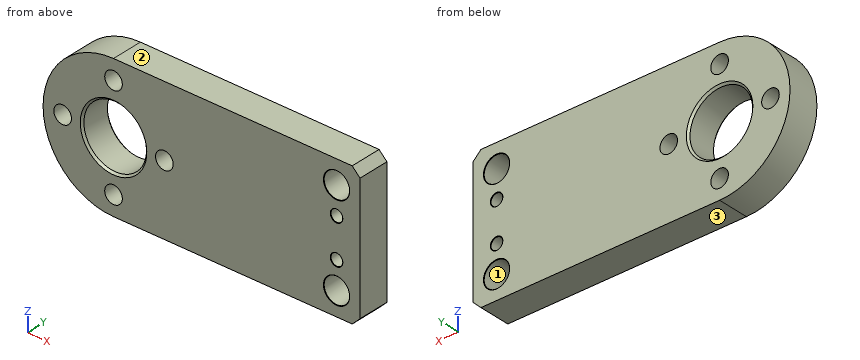
```python
from build123d import *

# Parameters (mm, degrees)
SKETCH1_R           = 8
SKETCH1_R_2         = 2.25
BOSS_EXTRUDE1_DEPTH = 8
SKETCH2_R           = 3.25
SKETCH2_R_2         = 1.5
CUT_EXTRUDE1_DEPTH  = 67.007575323
CHAMFER1_SIZE       = 0.5
CHAMFER2_SIZE       = 0.1


with BuildPart() as part:
    # Sketch1 → Boss-Extrude1 (new body)
    with BuildSketch(Plane(origin=(0, 0, 0), x_dir=(1, 0, 0), z_dir=(0, 1, 0))):
        with BuildLine():
            Line((0, 18), (61, 18))
            Line((61, 18), (63, 16))
            Line((63, 16), (63, -16))
            Line((63, -16), (61, -18))
            Line((61, -18), (0, -18))
            ThreePointArc((0, -18), (-18, 0), (0, 18))
        make_face()
        with Locations(Location((0, 0, 0), (0, 0, 270))):
            Circle(SKETCH1_R, mode=Mode.SUBTRACT)
        with Locations(Location((0, 13, 0), (0, 0, 270))):
            Circle(SKETCH1_R_2, mode=Mode.SUBTRACT)
        with Locations(Location((13, 0, 0), (0, 0, 270))):
            Circle(SKETCH1_R_2, mode=Mode.SUBTRACT)
        with Locations(Location((0, -13, 0), (0, 0, 270))):
            Circle(SKETCH1_R_2, mode=Mode.SUBTRACT)
        with Locations(Location((-13, 0, 0), (0, 0, 270))):
            Circle(SKETCH1_R_2, mode=Mode.SUBTRACT)
    extrude(amount=BOSS_EXTRUDE1_DEPTH)

    # Sketch2 → Cut-Extrude1 (cut, through all)
    with BuildSketch(Plane(origin=(0, 8, 0), x_dir=(1, 0, 0), z_dir=(0, 1, 0))):
        with Locations(Location((57, 12, 0), (0, 0, 270))):
            Circle(SKETCH2_R)
        with Locations(Location((57, 5, 0), (0, 0, 270))):
            Circle(SKETCH2_R_2)
        with Locations(Location((57, -5, 0), (0, 0, 90))):
            Circle(SKETCH2_R_2)
        with Locations(Location((57, -12, 0), (0, 0, 90))):
            Circle(SKETCH2_R)
    extrude(amount=-CUT_EXTRUDE1_DEPTH, mode=Mode.SUBTRACT)

    # Chamfer1
    chamfer1_edges = [part.edges().sort_by_distance(p)[0] for p in [
        (0, 0, -8),
        (0, 8, -8),
    ]]
    chamfer(chamfer1_edges, length=CHAMFER1_SIZE)

    # Chamfer2
    chamfer2_edges = [part.edges().sort_by_distance(p)[0] for p in [
        (57, 0, -15.25),
        (57, 8, -15.25),
        (57, 0, -6.5),
        (57, 8, -6.5),
        (57, 0, 6.5),
        (57, 8, 6.5),
        (57, 0, 15.25),
        (57, 8, 15.25),
    ]]
    chamfer(chamfer2_edges, length=CHAMFER2_SIZE)


solid = part.part
```
The listing builds one solid part. Answer for the finished solid, in the listing's coordinates (mm). Face numbers are marked on the shaded views. Give positions to 0.01 mm unless a question says otherwise; leave off trailing zeros. Order: outer loops, then holes, each group sorted by start corner. A loop starts at its lowest first (then second) coordinate and runs counter-clockwise, first axis right, second up. Notation, with made-up numbers: (49, 79.25) -> (100, 79.25) arc R32 ccw to (100, 108.25) -> close; hole circle Ø5 at (83.25, -10.75). An arc over 180 degrees is marked (long way). Write each question's results on one line, items separated by ' | '.
Q1. The part is cut by section C-C, the plane x = 13. Give the vertices of the cut face in (y, z).
Checked values:
outline: (0, -18) -> (8, -18) -> (8, -2.25) -> (0, -2.25) -> close; (0, 2.25) -> (8, 2.25) -> (8, 18) -> (0, 18) -> close
Q2. The part is cut by section B-B, the plane z = 0. Give the vertices of the cut face in (x, y).
Checked values:
outline: (-18, 0) -> (-15.25, 0) -> (-15.25, 8) -> (-18, 8) -> close; (-10.75, 0) -> (-8.5, 0) -> (-8, 0.5) -> (-8, 7.5) -> (-8.5, 8) -> (-10.75, 8) -> close; (8, 0.5) -> (8.5, 0) -> (10.75, 0) -> (10.75, 8) -> (8.5, 8) -> (8, 7.5) -> close; (15.25, 0) -> (63, 0) -> (63, 8) -> (15.25, 8) -> close
Q3. The part is cut by section D-D, the plane z = 12. Give the vertices of the cut face in (x, y), and give its area (3 significant figures).
Checked values:
outline: (-13.42, 0) -> (-2.02, 0) -> (-2.02, 8) -> (-13.42, 8) -> close; (2.02, 0) -> (53.65, 0) -> (53.75, 0.1) -> (53.75, 7.9) -> (53.65, 8) -> (2.02, 8) -> close; (60.25, 0.1) -> (60.35, 0) -> (63, 0) -> (63, 8) -> (60.35, 8) -> (60.25, 7.9) -> close | area: 527 mm^2
Q4. Each of these flat-tipped pins is pushed along its axis until it touches: P1, Ø9.5, axis at x = 0, z = 0, coming from the +Y side; P2, Ø4, axis at y = 5.5, z = 13.5, coming from the -X side. Where does it stop, or does it pass through?
Checked values:
P1: passes through | P2: stops at x = -13.85
Q5. Straight lines are drawn through the part: probe 1 along X at (y, z) = (4.5, 14); probe 2 along X at (y, z) = (4.25, -1.5); probe 3 along X at (y, z) = (3.5, -11). For each, find the intervals that lie inside material, in ascending order. Write a range as from..to.
Checked values:
probe 1: x = -11.31..-2.02, 2.02..54.44, 59.56..63 | probe 2: x = -17.94..-14.68, -11.32..-7.86, 7.86..11.32, 14.68..63 | probe 3: x = -14.25..-1.03, 1.03..53.91, 60.09..63
Q6. The part is cut by section A-A, the plane y = 4.5. State how many separate pieces and enclosed holes the cut face has, and give its area (3 significant figures).
Checked values:
separate pieces: 1 | enclosed holes: 9 | area: 2,430 mm^2
Q7. Determine the mould class of the marked faces 1, 2 and 3 for opening direction Z: pulls with the +Z half, pulls with the -Z half, needs draft (parallel to the pull), parting line crosses it, or undercut.
Checked values:
face 1: undercut | face 2: pulls with the +Z half | face 3: pulls with the -Z half
